```python
from build123d import *

# Parameters (mm, degrees)
F0_W      = 30
F0_H      = 30
F1_DEPTH  = 15
F2_R      = 4
F3_DEPTH  = 2
F4_R      = 4
F5_DEPTH  = 2
F7_DEPTH  = 2
F8_R      = 2
F10_DEPTH = 30


with BuildPart() as f1:
    # F0 (on Top) → F1 (new body, symmetric)
    with BuildSketch(Plane.XY):
        Rectangle(F0_W, F0_H)
    extrude(amount=F1_DEPTH, both=True)

    # F2 (on face) → F3 (cut)
    with BuildSketch(Plane.XY.offset(15)):
        Circle(F2_R)
    extrude(amount=-F3_DEPTH, mode=Mode.SUBTRACT)

    # F4 (on face) → F5 (cut)
    with BuildSketch(Plane.YZ.offset(15)):
        with Locations((-7, -7)):
            Circle(F4_R)
        with Locations((7, -7)):
            Circle(F4_R)
        with Locations((7, 7)):
            Circle(F4_R)
        with Locations((-7, 7)):
            Circle(F4_R)
    extrude(amount=-F5_DEPTH, mode=Mode.SUBTRACT)

    # F6 (on face) → F7 (cut)
    with BuildSketch(Plane.XZ.offset(15)):
        with BuildLine():
            ThreePointArc((-4.8005116586, 5.859375), (-4.6691210888, 6.4387772411), (-4.6249997839, 7.0312498137))
            ThreePointArc((-4.6249997839, 7.0312498137), (-12.0528271059, 9.0928025904), (-6.7499997094, 3.497926347))
            Line((-6.7499997094, 3.497926347), (-6.7499997094, 5.859375))
            Line((-6.7499997094, 5.859375), (-4.8005116586, 5.859375))
        make_face()
        with BuildLine():
            Line((-6.7499997094, 5.859375), (-6.7499997094, 3.497926347))
            ThreePointArc((-6.7499997094, 3.497926347), (-5.5403358849, 4.4847132187), (-4.8005116586, 5.859375))
            Line((-4.8005116586, 5.859375), (-6.7499997094, 5.859375))
        make_face()
        with BuildLine():
            ThreePointArc((-4.8005116586, 5.859375), (-5.5403358849, 4.4847132187), (-6.7499997094, 3.497926347))
            Line((-6.7499997094, 3.497926347), (-6.7499997094, -3.4687498119))
            Line((-6.7499997094, -3.4687498119), (2.6249999646, -3.4687498119))
            Line((2.6249999646, -3.4687498119), (2.6249999646, 5.859375))
            Line((2.6249999646, 5.859375), (-4.8005116586, 5.859375))
        make_face()
    extrude(amount=-F7_DEPTH, mode=Mode.SUBTRACT)

    # F8
    f8_edges = [f1.edges().sort_by_distance(p)[0] for p in [
        (0, -15, 15),
        (15, -15, 0),
        (15, 0, 15),
        (0, 15, 15),
        (-15, 0, 15),
        (-15, -15, 0),
        (0, -15, -15),
        (-15, 0, -15),
        (-15, 15, 0),
        (0, 15, -15),
        (15, 0, -15),
        (15, 15, 0),
    ]]
    fillet(f8_edges, radius=F8_R)

    # F9 (on face) → F10 (join)
    with BuildSketch(Plane(origin=(0, 0, -15), x_dir=(1, 0, 0), z_dir=(0, 0, -1))):
        with BuildLine():
            Line((-2.0403189119, 8.4453830495), (-9.9605508149, 8.4453830495))
            Line((-9.9605508149, 8.4453830495), (-9.9605508149, 0))
            Line((-9.9605508149, 0), (-5.5503539013, 0))
            ThreePointArc((-5.5503539013, 0), (-0.8939548861, -7.0463220271), (3.7624441291, 0))
            add(Edge.make_bspline(
                [(2.6284841664, 1.6503734824), (3.0064708206, 1.1002489883), (3.3844574749, 0.5501244941), (3.7624441291, 0)],
                knots=[8.2443845859, 8.2443845859, 8.2443845859, 8.2443845859, 10.2467826055, 10.2467826055, 10.2467826055, 10.2467826055], degree=3))
            add(Edge.make_bspline(
                [(-2.0403189119, 8.4453830495), (-0.4840512191, 6.1803798605), (1.0722164736, 3.9153766715), (2.6284841664, 1.6503734824)],
                knots=[0, 0, 0, 0, 8.2443845859, 8.2443845859, 8.2443845859, 8.2443845859], degree=3))
        make_face()
    extrude(amount=F10_DEPTH)


solid = f1.part
```
Here's how the part is built. I have some questions about the finished solid (model axes, mm). A direction names the side the tool comes from. Coordinates: 2 decimals unless noted, no trailing zeros. Order: outer loops, then holes, each group sorted by start corner. A loop starts at its lowest first (then second) coordinate and runs counter-clockwise, first axis right, second up. Notation, with made-up numbers: (-4, 31) - (7, 31) arc R17 ccw to (7, 39) - close; hole circle Ø8 at (-39, -9.5). An arc over 180 degrees is marked (long way). One line per question, with ' | ' between items. Start each with the question number.
1. Please list where these lines run through material, in increasing order: line 1 along Z through (x, y) = (13.55, 7); line 2 along Z through (x, y) = (13.9, -7); line 3 along Y through (x, z) = (-0.5, 5). Write a range as [from, to].
2. Which directions (+Z, -Z, +X, -X, +Y, -Y) give clear straight access to the entire face, cutting with the end or side of a thin tool? Please do faces 1 (the cylindrical face through (-0.867, -3.905, 14.014)), 2 (the flat face through (13, -7, -7)), 3 (the cylindrical face through (-14.43, 0.18, -14.4)).
3. If we section it at B-B (z = -7): Write out the boundary of the cut face in (x, y), and give its area (3 significant figures).
4. I'm going to push flat-ended pins straight in: pin 1 Ø4 at (x, y) = (8, 9) entering from -Z; pin 2 Ø9.5 at (y, z) = (-3, -29) entering from -X; pin 3 Ø5 at (y, z) = (-6, -26.5) entering from +X. Where does each tip first touch, or does it pass through?
5. If we mould it in two halves opening along Y, with no side actions, what happens to faces 4 (the flat face through (13, 7, -7)), 5 (the cylindrical face through (14.4, -14.43, 0.18)), 6 (the flat face through (-1, -14, 5.859))? For each: released by +Y, released by -Y, zero draft, split by the parting line, or undercut.
6. If we section it at A-A (x = 7.5): Write out the boundary of the cut face in (y, z), and give its area (3 significant figures).
7. If we section it at C-C (y = 2): Write out the boundary of the cut face in (x, z), and give its area (3 significant figures).
Model answer:
1) line 1: z = [-14.92, -11], [-3, 3], [11, 14.92] | line 2: z = [-14.79, -11], [-3, 3], [11, 14.79] | line 3: y = [-13, 15]
2) face 1: +Z | face 2: +X | face 3: -Z, -X, +Y, -Y
3) outline: (-15, -13) arc R2 ccw to (-13, -15) - (13, -15) arc R2 ccw to (15, -13) - (15, -11) - (13, -11) - (13, -3) - (15, -3) - (15, 3) - (13, 3) - (13, 11) - (15, 11) - (15, 13) arc R2 ccw to (13, 15) - (-13, 15) arc R2 ccw to (-15, 13) - close | area: 865 mm²
4) pin 1: stops at z = -15 | pin 2: stops at x = -9.96 | pin 3: stops at x = 1.36
5) face 4: undercut | face 5: released by -Y | face 6: zero draft
6) outline: (-15, -13) arc R2 ccw to (-13, -15) - (13, -15) arc R2 ccw to (15, -13) - (15, 13) arc R2 ccw to (13, 15) - (-13, 15) arc R2 ccw to (-15, 13) - close | area: 897 mm²
7) outline: (-15, -13) arc R2 ccw to (-13, -15) - (-5.96, -15) - (-5.96, -45) - (4.17, -45) - (4.17, -15) - (13, -15) arc R2 ccw to (15, -13) - (15, 13) arc R2 ccw to (13, 15) - (3.46, 15) - (3.46, 13) - (-3.46, 13) - (-3.46, 15) - (-13, 15) arc R2 ccw to (-15, 13) - close | area: 1,190 mm²
